The listing builds one solid part. Answer for the finished solid, in the listing's coordinates (mm). A direction names the side the tool comes from. Coordinates: 2 decimals unless noted, no trailing zeros. Order: outer loops, then holes, each group sorted by start corner. A loop starts at its lowest first (then second) coordinate and runs counter-clockwise, first axis right, second up. Notation, with made-up numbers: (18.5, 86) - (27.5, 86) arc R18 cw to (27.5, 97) - close; hole circle Ø4 at (57.5, -24). An arc over 180 degrees is marked (long way). Use one line per item in the form item = value. Start each with the question number.
Item 1: Each of these flat-tipped pins is pushed along its axis until it touches: pin 1 Ø1.5 at (x, z) = (7.5, 0) entering from -Y; pin 2 Ø1 at (x, z) = (-2.5, -4) entering from +Y; pin 3 Ø8 at (x, z) = (-15, 0) entering from +Y. Where does it stop, or does it pass through?
Item 2: A tool of negligible diameter and unlimited length cuts with its end or side. For faces 1 (the flat face through (-9.4, 0.7, 6.4)), 2 (the cylindrical face through (-7.37, 3.39, -1.64)), from which of +Z, -Z, +X, -X, +Y, -Y can it reach the whole face along a straight path? Write none if from no direction.
Item 3: Consider line 1 along X through (y, z) = (1.25, 0.5); line 2 along Y through (x, z) = (-17, 3); line 3 along Z through (x, y) = (-2, 0.85). Determine where each line is inside the solid, lowest interval first. Write a range as [from, to].
Item 4: The mould has two halves that part along X. Classify faces 3 (the flat face through (9.4, 0.7, -6.4)), 4 (the cylindrical face through (0.9, 1.11, 2.86)), 5 (the flat face through (12.6, 1.5, -0.1)): released by +X, released by -X, zero draft, split by the parting line, or undercut.
Item 5: Section D-D, the plane x = -15 is taken. Write down the section's boundary in (y, z), and give its area (3 significant figures).
Item 6: Section B-B, the plane y = 2.7 is taken. Write down the section's boundary in (x, z), and give its area (3 significant figures).
Item 7: Section A-A, the plane x = 0 is taken. Write down the section's boundary in (y, z).
Item 8: Section C-C, the plane z = -3.75 is taken. Write down the section's boundary in (x, y).
from build123d import *
from build123d.topology import SkipClean

# Parameters (mm, degrees)
SKETCH1_R           = 1.5
SKETCH1_R_2         = 3
BOSS_EXTRUDE1_DEPTH = 4.4972
CUT_EXTRUDE2_START  = 4.4972
SKETCH1_6_R         = 7.55
CUT_EXTRUDE2_DEPTH  = 2.25
CUT_EXTRUDE1_START  = 1.5
SKETCH1_5_R         = 1.5
CUT_EXTRUDE1_DEPTH  = 2.9972


with BuildPart() as part:
    # Sketch1 → Boss-Extrude1 (new body)
    with BuildSketch(Plane(origin=(0, 0, 0), x_dir=(1, 0, 0), z_dir=(0, 1, 0))):
        with BuildLine():
            Line((15.901070321, 4.277965365), (2.792140641, 8.555930729))
            ThreePointArc((2.792140641, 8.555930729), (0, 9), (-2.792140641, 8.555930729))
            Line((-2.792140641, 8.555930729), (-15.901070321, 4.277965365))
            ThreePointArc((-15.901070321, 4.277965365), (-19.005, 0), (-15.901070321, -4.277965365))
            Line((-15.901070321, -4.277965365), (-2.792140641, -8.555930729))
            ThreePointArc((-2.792140641, -8.555930729), (0, -9), (2.792140641, -8.555930729))
            Line((2.792140641, -8.555930729), (15.901070321, -4.277965365))
            ThreePointArc((15.901070321, -4.277965365), (19.005, 0), (15.901070321, 4.277965365))
        make_face()
        with Locations(Location((14.505, 0, 0), (0, 0, 270))):
            Circle(SKETCH1_R, mode=Mode.SUBTRACT)
        with Locations(Location((-14.505, 0, 0), (0, 0, 270))):
            Circle(SKETCH1_R, mode=Mode.SUBTRACT)
        with Locations(Location((0, 0, 0), (0, 0, 270))):
            Circle(SKETCH1_R_2, mode=Mode.SUBTRACT)
    extrude(amount=BOSS_EXTRUDE1_DEPTH)

    # Sketch1<6> → Cut-Extrude2 (cut)
    with BuildSketch(Plane(origin=(0, 0, 0), x_dir=(1, 0, 0), z_dir=(0, 1, 0)).offset(CUT_EXTRUDE2_START)):
        with Locations(Location((0, 0, 0), (0, 0, 270))):
            Circle(SKETCH1_6_R)
    extrude(amount=-CUT_EXTRUDE2_DEPTH, mode=Mode.SUBTRACT)

    # Sketch1<5> → Cut-Extrude1 (cut)
    # profile 1 of 2: a face of its own
    with SkipClean():  # the faces are left unmerged after this step: merging them gives an invalid solid
        with BuildSketch(Plane(origin=(0, 0, 0), x_dir=(1, 0, 0), z_dir=(0, 1, 0)).offset(CUT_EXTRUDE1_START)):
            with BuildLine():
                Line((-15.901070321, -4.277965365), (-2.792140641, -8.555930729))
                ThreePointArc((-2.792140641, -8.555930729), (-9, 0), (-2.792140641, 8.555930729))
                Line((-2.792140641, 8.555930729), (-15.901070321, 4.277965365))
                ThreePointArc((-15.901070321, 4.277965365), (-19.005, 0), (-15.901070321, -4.277965365))
            make_face()
            with Locations(Location((-14.505, 0, 0), (0, 0, 270))):
                Circle(SKETCH1_5_R, mode=Mode.SUBTRACT)
        # profile 2 of 2: a face of its own
        with BuildSketch(Plane(origin=(0, 0, 0), x_dir=(1, 0, 0), z_dir=(0, 1, 0)).offset(CUT_EXTRUDE1_START)):
            with BuildLine():
                ThreePointArc((9, 0), (7.284547542, -5.28539186), (2.792140641, -8.555930729))
                Line((2.792140641, -8.555930729), (15.901070321, -4.277965365))
                ThreePointArc((15.901070321, -4.277965365), (19.005, 0), (15.901070321, 4.277965365))
                Line((15.901070321, 4.277965365), (2.792140641, 8.555930729))
                ThreePointArc((2.792140641, 8.555930729), (7.284547542, 5.28539186), (9, 0))
            make_face()
            with Locations(Location((14.505, 0, 0), (0, 0, 270))):
                Circle(SKETCH1_5_R, mode=Mode.SUBTRACT)
        extrude(amount=CUT_EXTRUDE1_DEPTH, mode=Mode.SUBTRACT)


solid = part.part
Response:
q1.pin_1 = 0
q1.pin_2 = 2.25
q1.pin_3 = 1.5
q2.face_1 = +Z, -X, +Y, -Y
q2.face_2 = +Y
q3.line_1 = [-18.98, -15.92], [-13.09, -2.96], [2.96, 13.09], [15.92, 18.98]
q3.line_2 = [0, 1.5]
q3.line_3 = [-8.77, -2.24], [2.24, 8.77]
q4.face_3 = released by +X
q4.face_4 = undercut
q4.face_5 = zero draft
q5.outline = (0, -4.57) - (1.5, -4.57) - (1.5, -1.42) - (0, -1.42) - close; (0, 1.42) - (1.5, 1.42) - (1.5, 4.57) - (0, 4.57) - close
q5.area = 9.47 mm2
q6.outline = circle Ø18 at (0, 0); hole circle Ø15.1 at (0, 0)
q6.area = 75.4 mm2
q7.outline = (0, -9) - (4.5, -9) - (4.5, -7.55) - (2.25, -7.55) - (2.25, -3) - (0, -3) - close; (0, 3) - (2.25, 3) - (2.25, 7.55) - (4.5, 7.55) - (4.5, 9) - (0, 9) - close
q8.outline = (-16.99, 0) - (16.99, 0) - (16.99, 1.5) - (8.18, 1.5) - (8.18, 4.5) - (6.55, 4.5) - (6.55, 2.25) - (-6.55, 2.25) - (-6.55, 4.5) - (-8.18, 4.5) - (-8.18, 1.5) - (-16.99, 1.5) - close
